from build123d import *

# Parameters (mm, degrees)
SKETCH_1_W          = 22
SKETCH_1_H          = 17
EXTRUDE_1_DEPTH     = 11
SKETCH_3_W          = 10
SKETCH_3_H          = 17.5
EXTRUDE_2_DEPTH     = 9
SKETCH_4_R          = 1.6
CUT_EXTRUDE_1_DEPTH = 22
SKETCH_5_W          = 8
SKETCH_5_H          = 8
CUT_EXTRUDE_2_DEPTH = 22
FILLET_1_R          = 1.5
FILLET_START        = -6
FILLET_2_DEPTH      = 11
FILLET_START_2      = -5
FILLET_2_2_DEPTH    = 10
SKETCH_7_W          = 37.569031752
SKETCH_7_H          = 53.082934042
CUT_EXTRUDE_4_DEPTH = 22
SKETCH_8_R          = 1
CUT_EXTRUDE_5_DEPTH = 1.5


with BuildPart() as part:
    # 草图1 → 凸台-拉伸1 (new, symmetric)
    with BuildSketch(Plane.XY):
        with Locations((0, -2.5)):
            Rectangle(SKETCH_1_W, SKETCH_1_H)
    extrude(amount=EXTRUDE_1_DEPTH, both=True)

    # 草图2 → 切除-旋转1 (revolve, cut)
    with BuildSketch(Plane.XY, mode=Mode.PRIVATE) as cut_revolve_1_sk:
        with BuildLine():
            Line((0, 6), (6.708203932, 6))
            ThreePointArc((6.708203932, 6), (8.215838363, -3.674234614), (0, -9))
            Line((0, -9), (0, 6))
        make_face()
    revolve(cut_revolve_1_sk.sketch.rotate(Axis((0, 0, 0), (0, 1, 0)), 180), axis=Axis((0, 0, 0), (0, 1, 0)), mode=Mode.SUBTRACT)

    # 草图3 → 凸台-拉伸2 (add, symmetric)
    with BuildSketch(Plane.XY):
        with Locations((0, 14.75)):
            Rectangle(SKETCH_3_W, SKETCH_3_H)
    extrude(amount=EXTRUDE_2_DEPTH, both=True)

    # 草图4 → 切除-拉伸1 (cut)
    with BuildSketch(Plane(origin=(0, 23.5, 0), x_dir=(1, 0, 0), z_dir=(0, 1, 0))):
        with Locations(Location((0, 0, 0), (0, 0, 180))):
            Circle(SKETCH_4_R)
    extrude(amount=-CUT_EXTRUDE_1_DEPTH, mode=Mode.SUBTRACT)

    # 草图5 → 切除-拉伸2 (cut)
    with BuildSketch(Plane.ZY.offset(5)):
        with Locations((0, 10)):
            Rectangle(SKETCH_5_W, SKETCH_5_H)
    extrude(amount=-CUT_EXTRUDE_2_DEPTH, mode=Mode.SUBTRACT)

    # 圆角1
    fillet_1_edges = [part.edges().sort_by_distance(p)[0] for p in [
        (0, -11, 11),
        (11, -2.5, 11),
        (5, 14.75, -9),
        (0, 23.5, -9),
        (5, 23.5, 0),
        (-5, 14.75, -9),
        (-5, 23.5, 0),
        (5, 14.75, 9),
        (0, 23.5, 9),
        (-5, 14.75, 9),
        (0, 6, 11),
        (11, -2.5, -11),
        (0, -11, -11),
        (-11, -2.5, -11),
        (0, 6, -11),
        (11, 6, 0),
        (11, -11, 0),
        (-11, -11, 0),
        (-11, 6, 0),
        (-11, -2.5, 11),
    ]]
    fillet(fillet_1_edges, radius=FILLET_1_R)

    # 圆角2: read off the stored shape, not the designer's step
    # 圆角2 outline → 圆角2 (cut)
    with BuildSketch(Plane.YZ.offset(FILLET_START)):
        with BuildLine():
            Line((6, -4), (6, -5.5))
            ThreePointArc((6, -5.5), (6.439339828, -4.439339828), (7.5, -4))
            Line((7.5, -4), (6, -4))
        make_face()
        with BuildLine():
            Line((6, 4), (7.5, 4))
            ThreePointArc((7.5, 4), (6.439339828, 4.439339828), (6, 5.5))
            Line((6, 5.5), (6, 4))
        make_face()
    extrude(amount=FILLET_2_DEPTH, mode=Mode.SUBTRACT)

    # Fillet 2 2 outline → Fillet 2 2 (add)
    with BuildSketch(Plane.YZ.offset(FILLET_START_2)):
        with BuildLine():
            ThreePointArc((12.5, 4), (13.560660172, 3.560660172), (14, 2.5))
            Line((14, 2.5), (14, 4))
            Line((14, 4), (12.5, 4))
        make_face()
        with BuildLine():
            ThreePointArc((14, -2.5), (13.560660172, -3.560660172), (12.5, -4))
            Line((12.5, -4), (14, -4))
            Line((14, -4), (14, -2.5))
        make_face()
    extrude(amount=FILLET_2_2_DEPTH)

    # 草图7 → 切除-拉伸4 (cut)
    with BuildSketch(Plane(origin=(0, 0, 0), x_dir=(0, 0, -1), z_dir=(1, 0, 0))):
        Rectangle(SKETCH_7_W, SKETCH_7_H)
    extrude(amount=-CUT_EXTRUDE_4_DEPTH, mode=Mode.SUBTRACT)

    # 草图8 → 切除-拉伸5 (cut)
    with BuildSketch(Plane.ZY):
        with Locations((6, 20.5)):
            Circle(SKETCH_8_R)
        with Locations((8.5, -8.5)):
            Circle(SKETCH_8_R)
        with Locations(Location((-6, 20.5, 0), (0, 0, 180))):
            Circle(SKETCH_8_R)
        with Locations(Location((-8.5, -8.5, 0), (0, 0, 180))):
            Circle(SKETCH_8_R)
    extrude(amount=-CUT_EXTRUDE_5_DEPTH, mode=Mode.SUBTRACT)


solid = part.part
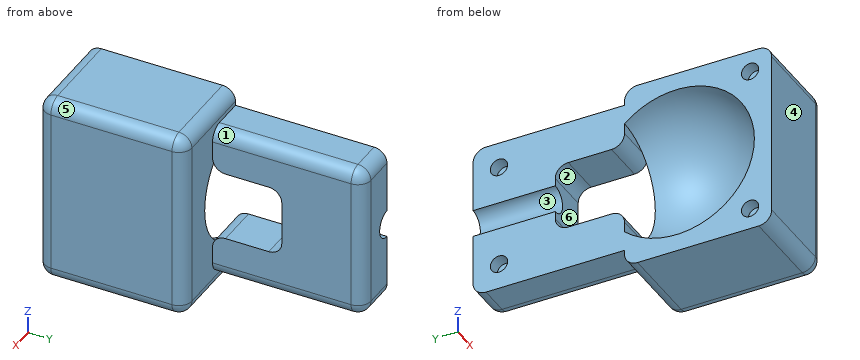
Design review of the part built by this model. Coordinates are the model's own, in mm. Face numbers are marked on the shaded views. A direction names the side the tool comes from. Round coordinates to 2 decimals unless told otherwise and drop trailing zeros. Write each loop counter-clockwise with the first axis right and the second up, starting at its lowest first coordinate (ties: lowest second). Pieces come first, ordered by that corner, then holes. Notation, with made-up numbers: (14.5, 43.25) - (24.5, 43.25) arc R22 ccw to (24.5, 69.25) - close; hole circle Ø9 at (48.25, 35). An arc over 180 degrees is marked (long way). Use a Markdown table: item, result. Add a question column.
1. Mouldability with a two-part tool opening along Y and no side actions: class the marked faces 4, 5 and 6 as +Y half, -Y half, draft (parallel to the pull), parting line (faces both ways), or undercut.
2. We need section A-A (y = 8). State the section outline as (x, z) points.
3. We need section D-D (x = 8.5). State the section outline as (y, z) points, then the cut area to 3 significant figures.
4. Wall thickness on probe 1 along Y at (x, z) = (0.4, -6); probe 2 along X at (y, z) = (17, -4.75); probe 3 along Y at (x, z) = (8, -7): over which ranges is each line inside the solid? List them lowest first.
5. Clearance check with flat-ended pins moving along their axes: pin 1 (6 mm diameter, centred on x = 9, z = -0.5, fed in from +Y); pin 2 (1.5 mm diameter, centred on x = 3, y = 9.5, fed in from +Z); pin 3 (1.5 mm diameter, centred on x = 3.5, y = 10.5, fed in from -Z). State where each tip first meets the part, or that it passes through.
6. We need section C-C (z = 6). State the section outline as (x, y) points, then the cut area to 3 significant figures.
7. We need section B-B (z = 0). State the section outline as (x, y) points.
8. For the marked faces 1, 2 and 3, list the 3-axis set-ups (+Z, -Z, +X, -X, +Y, -Y) from which the entire face can be reached by the end or side of a thin tool; tool diameter is ignored.
Output:
| question | item | result |
|---|---|---|
| 1 | face 4 | -Y half |
| 1 | face 5 | draft |
| 1 | face 6 | undercut |
| 2 | outline | (0, -9) - (3.5, -9) arc R1.5 ccw to (5, -7.5) - (5, -4) - (0, -4) - close; (0, 4) - (5, 4) - (5, 7.5) arc R1.5 ccw to (3.5, 9) - (0, 9) - close |
| 3 | outline | (-11, -9.5) arc R1.5 ccw to (-9.5, -11) - (4.5, -11) arc R1.5 ccw to (6, -9.5) - (6, 9.5) arc R1.5 ccw to (4.5, 11) - (-9.5, 11) arc R1.5 ccw to (-11, 9.5) - close; hole circle Ø5.92 at (0, 0) |
| 3 | area | 345 mm2 |
| 4 | probe 1 | y = -11 to -6.7, 6 to 19.5, 21.5 to 23.5 |
| 4 | probe 2 | x = 0 to 5 |
| 4 | probe 3 | y = -11 to 6 |
| 5 | pin 1 | stops at y = 6 |
| 5 | pin 2 | stops at z = 9 |
| 5 | pin 3 | stops at z = -9 |
| 6 | outline | (0, -11) - (9.5, -11) arc R1.5 ccw to (11, -9.5) - (11, 4.5) arc R1.5 ccw to (9.5, 6) - (5, 6) - (5, 22) arc R1.5 ccw to (3.5, 23.5) - (0, 23.5) - (0, 21.5) - (1.5, 21.5) - (1.5, 19.5) - (0, 19.5) - (0, 6) - (3, 6) arc R6.71 cw to (0, -6.71) - close |
| 6 | area | 201 mm2 |
| 7 | outline | (0, -11) - (9.5, -11) arc R1.5 ccw to (11, -9.5) - (11, 4.5) arc R1.5 ccw to (9.5, 6) - (6.71, 6) arc R9 cw to (0, -9) - close; (1.6, 14) - (5, 14) - (5, 22) arc R1.5 ccw to (3.5, 23.5) - (1.6, 23.5) - close |
| 8 | face 1 | +Z, +X, +Y |
| 8 | face 2 | +X, -X |
| 8 | face 3 | -X, +Y |
